```python
from build123d import *

# Parameters (mm, degrees)
F1_W = 3.683
F1_H = 3.683
F1_R = 1.5875
F3_R = 1.84149


# Not quite as in the source:
# - a fillet or chamfer is up to 0.001 mm smaller than in the source, because OpenCascade refuses the exact size


with BuildPart() as f2:
    # F2: sweep along a path in F0
    with BuildLine(Plane.XY) as f2_path:
        Line((0, 0), (0, -3.175))
        ThreePointArc((0, -3.175), (-2.8623663141, -7.3624320102), (-7.8033180665, -6.2158180665))
        ThreePointArc((-7.8033180665, -6.2158180665), (-9.3053739342, -5.1418390585), (-11.1125, -4.7625))
        Line((-11.1125, -4.7625), (-14.2875, -4.7625))
    # F1 (on Front) → F2 (sweep)
    with BuildSketch(Plane.XZ):
        Rectangle(F1_W, F1_H)
        Circle(F1_R, mode=Mode.SUBTRACT)
    sweep(path=f2_path.line)

    # F3 (radius 1.8415 in the source; OpenCascade refuses exactly that, so slightly less here)
    f3_edges = [f2.edges().sort_by_distance(p)[0] for p in [
        (-12.7, -6.604, -1.8415),
        (-12.7, -6.604, 1.8415),
        (-12.7, -2.921, 1.8415),
        (-12.7, -2.921, -1.8415),
    ]]
    fillet(f3_edges, radius=F3_R)


solid = f2.part
```
Model file for the job. Use its own axes, mm. A direction names the side the tool comes from. Coordinates: 2 decimals unless noted, no trailing zeros. Write each loop counter-clockwise with the first axis right and the second up, starting at its lowest first coordinate (ties: lowest second). Pieces come first, ordered by that corner, then holes. Notation, with made-up numbers: (73, 58.5) - (123, 58.5) arc R23 ccw to (123, 92.5) - close; hole circle Ø2 at (-37.75, 46). An arc over 180 degrees is marked (long way). One line per question, with ' | ' between items. Start each with the question number.
Q1. Pin check, flat tips, straight feed: pin 1 (4 mm diameter, centred on x = -4.5, y = -5, fed in from -Z); pin 2 (1 mm diameter, centred on x = -3.5, z = 1, fed in from +Y); pin 3 (1.5 mm diameter, centred on x = -3.5, y = -3.5, fed in from +Z); pin 4 (1.5 mm diameter, centred on y = -4, z = 0.5, fed in from +X). Stop position of each tip, or through.
Q2. Drill centre lines: line 1 (Z direction, x = 0, y = -1.35); line 2 (X direction, y = -4.25, z = 0.3); line 3 (X direction, y = -0.75, z = -0.7). Where is each one in solid material? Low to high. Write a range as [from, to].
Q3. 3-axis set-ups, long thin cutter, end or side, ignore diameter. For faces 1 (the face through (-12.722, -6.05, -1.316)), 2 (the face through (-12.72, -6.23, -0.61)), 3 (the face through (-12.722, -6.05, 1.316)): which of +Z, -Z, +X, -X, +Y, -Y reach the whole face in a straight line?
Q4. Pull direction X, two halves, no side cores. Call faces 4 (the face through (1.288, -1.61, 1.316)), 5 (the face through (-12.722, -3.475, -1.316)), 6 (the face through (-0.34, -1.61, -1.55)): pulls with the +X half, pulls with the -X half, needs draft (parallel to the pull), parting line crosses it, or undercut.
Q5. Cut at D-D, the plane z = -1.4. List the corners of the cut face in (x, y) (1 decimal).
Answer below:
1) pin 1: z = -1.72 | pin 2: y = -5.59 | pin 3: through | pin 4: x = 1.84
2) line 1: [-1.84, -1.59], [1.59, 1.84] | line 2: [-7.71, -7.27], [-2.04, -1.76], [1.46, 1.72] | line 3: [-1.7, -1.42], [1.42, 1.7]
3) face 1: -Z, -X, -Y | face 2: -X | face 3: +Z, -X, -Y
4) face 4: pulls with the +X half | face 5: needs draft | face 6: undercut
5) outline: (-14.3, -6) - (-11.1, -6) arc R3.3 cw to (-8.7, -7) arc R5.7 ccw to (1.2, -3.2) - (1.2, 0) - (0.7, 0) - (0.7, -3.2) arc R5.2 cw to (-8.4, -6.7) arc R3.7 ccw to (-11.1, -5.5) - (-14.3, -5.5) - close; (-14.3, -4) - (-11.1, -4) arc R5.2 cw to (-7.3, -5.7) arc R3.7 ccw to (-0.7, -3.2) - (-0.7, 0) - (-1.2, 0) - (-1.2, -3.2) arc R3.3 cw to (-6.9, -5.4) arc R5.7 ccw to (-11.1, -3.6) - (-14.3, -3.6) - close
